from build123d import *

# Parameters (mm, degrees)
ESQUISSE1_W                  = 15
ESQUISSE1_H                  = 30
BOSS_EXTRU_1_DEPTH           = 3
ESQUISSE2_R                  = 1.5
ENL_V_MAT_EXTRU_2_DEPTH      = 3
ESQUISSE3_R                  = 3.5
ENL_V_MAT_EXTRU_3_DEPTH      = 2
ESQUISSE4_R                  = 3
BOSS_EXTRU_2_DEPTH           = 5.2
CONG_3_R                     = 2
CONG_4_R                     = 1
ESQUISSE5_R                  = 1.5
ENL_V_MAT_EXTRU_4_DEPTH      = 18
ENL_V_MAT_EXTRU_4_DEPTH_BACK = 18
CHANFREIN2_SIZE              = 0.2


with BuildPart() as part:
    # Esquisse1 → Boss.-Extru.1 (new body)
    with BuildSketch(Plane.XY):
        with Locations((7.5, 15)):
            Rectangle(ESQUISSE1_W, ESQUISSE1_H)
    extrude(amount=BOSS_EXTRU_1_DEPTH)

    # Esquisse2 → Enlèv. mat.-Extru.2 (cut)
    with BuildSketch(Plane.XY):
        with Locations((7.5, 25)):
            Circle(ESQUISSE2_R)
        with Locations((7.5, 5)):
            Circle(ESQUISSE2_R)
    extrude(amount=ENL_V_MAT_EXTRU_2_DEPTH, mode=Mode.SUBTRACT)

    # Esquisse3 → Enlèv. mat.-Extru.3 (cut)
    with BuildSketch(Plane.XY):
        with Locations((7.5, 25)):
            Circle(ESQUISSE3_R)
        with Locations((7.5, 5)):
            Circle(ESQUISSE3_R)
    extrude(amount=ENL_V_MAT_EXTRU_3_DEPTH, mode=Mode.SUBTRACT)

    # Esquisse4 → Boss.-Extru.2 (add)
    with BuildSketch(Plane.XY):
        with Locations((7.5, 13)):
            Circle(ESQUISSE4_R)
    extrude(amount=-BOSS_EXTRU_2_DEPTH)

    # Congé3
    cong_3_edges = [part.edges().sort_by_distance(p)[0] for p in [
        (0, 30, 1.5),
        (15, 30, 1.5),
        (15, 0, 1.5),
        (0, 0, 1.5),
    ]]
    fillet(cong_3_edges, radius=CONG_3_R)

    # Congé4
    cong_4_edges = [part.edges().sort_by_distance(p)[0] for p in [
        (7.5, 30, 0),
        (0, 15, 0),
        (15, 15, 0),
        (7.5, 0, 0),
        (0.585786438, 29.414213562, 0),
        (0.585786438, 0.585786438, 0),
        (14.414213562, 0.585786438, 0),
        (14.414213562, 29.414213562, 0),
    ]]
    fillet(cong_4_edges, radius=CONG_4_R)

    # Esquisse5 → Enlèv. mat.-Extru.4 (cut, two sides)
    with BuildSketch(Plane.XY) as enl_v_mat_extru_4_sk:
        with Locations((7.5, 13)):
            Circle(ESQUISSE5_R)
    extrude(amount=ENL_V_MAT_EXTRU_4_DEPTH, mode=Mode.SUBTRACT)
    extrude(enl_v_mat_extru_4_sk.sketch, amount=-ENL_V_MAT_EXTRU_4_DEPTH_BACK, mode=Mode.SUBTRACT)

    # Chanfrein2
    chanfrein2_edges = [part.edges().sort_by_distance(p)[0] for p in [
        (4.5, 13, -5.2),
    ]]
    chamfer(chanfrein2_edges, length=CHANFREIN2_SIZE)


solid = part.part
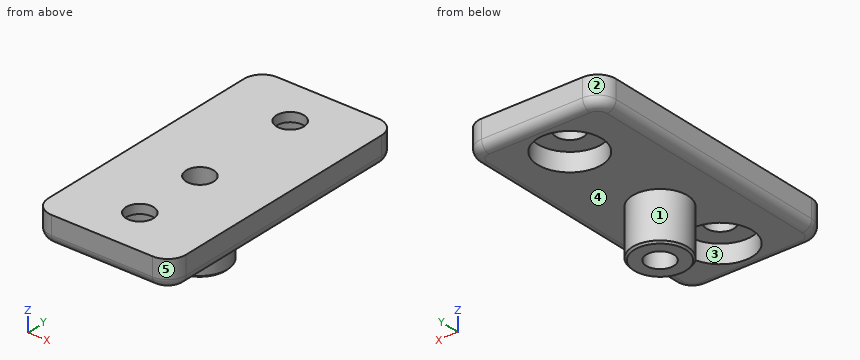
Could you check a few things on this model? Use its own coordinates, in mm. Face numbers are marked on the shaded views. A direction names the side the tool comes from. Give positions to 0.01 mm unless a question says otherwise; leave off trailing zeros. Order: outer loops, then holes, each group sorted by start corner. A loop starts at its lowest first (then second) coordinate and runs counter-clockwise, first axis right, second up. Notation, with made-up numbers: (39, 60) - (45, 60) arc R14 cw to (45, 77) - close; hole circle Ø9 at (12.5, 78). An arc over 180 degrees is marked (long way). One line per question, with ' | ' between items. Start each with the question number.
Item 1: I want a section at B-B on x = 3. Write out the boundary of the cut face in (y, z), then the cut area to 3 significant figures.
Item 2: Thinking about a two-plate mould opening in Y: for the marked faces 3, 4 and 5, which applies, pulls with the +Y half, pulls with the -Y half, needs draft (parallel to the pull), parting line crosses it, or undercut?
Item 3: I'm going to push flat-ended pins straight in: pin 1 Ø1 at (x, y) = (9.5, 24.5) entering from -Z; pin 2 Ø3.5 at (x, y) = (7.5, 25) entering from +Z; pin 3 Ø7.5 at (x, y) = (7, 26.5) entering from -Z; pin 4 Ø1.5 at (x, z) = (6, -3.5) entering from +Y. Where does each tip first touch, or does it pass through?
Item 4: I want a section at D-D on z = -2. Write out the boundary of the cut face in (x, y), then the cut area to 3 significant figures.
Item 5: I want a section at A-A on y = 25. Write out the boundary of the cut face in (x, z), then the cut area to 3 significant figures.
Item 6: For the marked faces 1 and 2, which set-ups out of +Z, -Z, +X, -X, +Y, -Y let a thin tool reach every point of the face, with its end or its side?
Item 7: I need wall thicknesses on probe 1 along Y at (x, z) = (7.5, 2.5); probe 2 along Y at (x, z) = (6.75, 2.25); probe 3 along X at (y, z) = (5, 2.35). Which ranges of each line are inside material? Lowest first, please. Write a range as [from, to].
Item 8: I want a section at C-C on y = 9.5. Write out the boundary of the cut face in (x, z).
Verdict:
1) outline: (0, 1) arc R1 ccw to (1, 0) - (29, 0) arc R1 ccw to (30, 1) - (30, 3) - (0, 3) - close | area: 89.6 mm^2
2) face 3: undercut | face 4: needs draft | face 5: pulls with the -Y half
3) pin 1: z = 2 | pin 2: z = 3 | pin 3: z = 0 | pin 4: y = 15.9
4) outline: circle Ø6 at (7.5, 13); hole circle Ø3 at (7.5, 13) | area: 21.2 mm^2
5) outline: (0, 1) arc R1 ccw to (1, 0) - (4, 0) - (4, 2) - (6, 2) - (6, 3) - (0, 3) - close; (9, 2) - (11, 2) - (11, 0) - (14, 0) arc R1 ccw to (15, 1) - (15, 3) - (9, 3) - close | area: 27.6 mm^2
6) face 1: -Z | face 2: +Z, -Z, -X, +Y
7) probe 1: [0, 3.5], [6.5, 11.5], [14.5, 23.5], [26.5, 30] | probe 2: [0, 3.7], [6.3, 11.7], [14.3, 23.7], [26.3, 30] | probe 3: [0, 6], [9, 15]
8) outline: (0, 1) arc R1 ccw to (1, 0) - (14, 0) arc R1 ccw to (15, 1) - (15, 3) - (0, 3) - close
